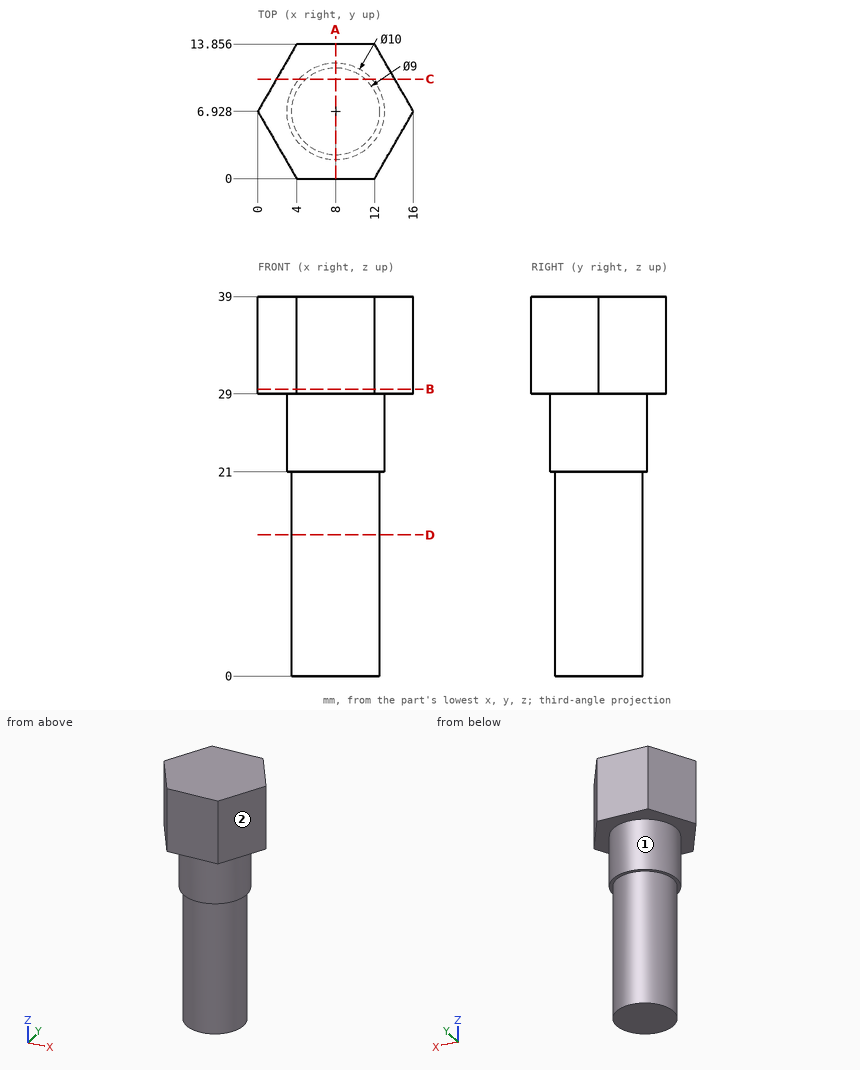
Answer from the drawing. Dimensions are ordinates in mm from the lowest x, y and z of the part. A direction names the side the tool comes from. Coordinates: 2 decimals unless noted, no trailing zeros. Order: outer loops, then holes, each group sorted by start corner. A loop starts at its lowest first (then second) coordinate and runs counter-clockwise, first axis right, second up. Notation, with made-up numbers: (17, 39) - (65, 39) arc R36 ccw to (65, 76) - close; hole circle Ø2 at (9.25, 54). An arc over 180 degrees is marked (long way). Answer as a JSON object with one key per item and string values. Group by question number.
Item 1: Section A-A (x = 8) is taken. Give the vertices of the cut face in (y, z).
Item 2: Section D-D (z = 14.5) is taken. Give the vertices of the cut face in (x, y).
Item 3: Flat-ended cylindrical pins translate along their axes: P1, Ø1, axis at y = 4, z = 27.5, coming from the +X side; P2, Ø3, axis at x = 10, y = 5, coming from the -Z side; P3, Ø5, axis at x = 3.5, z = 8, coming from the -Y side; P4, Ø2, axis at x = 11.5, z = 20.5, coming from the +Y side. Find the tip coordinate at first contact, or state that the pin passes through.
Item 4: A tool of negligible diameter and unlimited length cuts with its end or side. For the marked faces 1 and 2, from which of +Z, -Z, +X, -X, +Y, -Y can it reach the whole face along a straight path? Write none if from no direction.
Item 5: Section B-B (z = 29.5) is taken. Give the vertices of the cut face in (x, y).
Item 6: Section C-C (y = 10.25) is taken. Give the vertices of the cut face in (x, z) (1 decimal).
Item 7: Consider probe 1 along Z at (x, y) = (7.5, 13.5); probe 2 along X at (y, z) = (7, 15.5); probe 3 along Z at (x, y) = (3.5, 6). Determine where each line is inside the solid, lowest interval first. Write a range as from..to.
Results are:
{
 "1": {"outline": "(0, 29) - (1.93, 29) - (1.93, 21) - (2.43, 21) - (2.43, 0) - (11.43, 0) - (11.43, 21) - (11.93, 21) - (11.93, 29) - (13.86, 29) - (13.86, 39) - (0, 39) - close"},
 "2": {"outline": "circle Ø9 at (8, 6.93)"},
 "3": {"P1": "stops at x = 12.37", "P2": "stops at z = 0", "P3": "stops at y = 2.9", "P4": "stops at y = 11.18"},
 "4": {"face 1": "-Z", "face 2": "+Z, -Z, +X, -Y"},
 "5": {"outline": "(0, 6.93) - (4, 0) - (12, 0) - (16, 6.93) - (12, 13.86) - (4, 13.86) - close"},
 "6": {"outline": "(1.9, 29) - (4.3, 29) - (4.3, 21) - (5, 21) - (5, 0) - (11, 0) - (11, 21) - (11.7, 21) - (11.7, 29) - (14.1, 29) - (14.1, 39) - (1.9, 39) - close"},
 "7": {"probe 1": "z = 29..39", "probe 2": "x = 3.5..12.5", "probe 3": "z = 21..39"}
}
